Geometry check sheet. Reference: the model listing, model coordinates, mm. Give positions to 0.01 mm unless a question says otherwise; leave off trailing zeros. Write each loop counter-clockwise with the first axis right and the second up, starting at its lowest first coordinate (ties: lowest second). Pieces come first, ordered by that corner, then holes. Notation, with made-up numbers: M 0.25,10 L 40.25,10 A26 ccw 40.25,35 Z; hole C 76.25,43 d4. An arc over 180 degrees is marked long. Use one line per item in the form item = value. Start each with the question number.
Autodesk Inventor part; units mm, degrees
ref_plane "作業平面1" through (0, 0, 0) normal (0, 0, -1) x (-1, 0, 0)
ref_plane "YZ Plane" through (0, 0, 0) normal (1, 0, 0) x (0, 1, 0)
ref_plane "XZ Plane" through (0, 0, 0) normal (0, 1, 0) x (-1, 0, 0)
sketch "スケッチ1" plane through (0, 0, 0) normal (0, 0, 1) x (1, 0, 0)
  circle A0 centre (0, 0) radius 5
  circle A1 centre (0, 0) radius 4.5
  dimension "d0" = 10
  dimension "d10" = 9
ref_plane "作業平面1" through (0, 0, 0) normal (0, 0, -1) x (-1, 0, 0)
extrude "押し出し5" add sketch "スケッチ1" against normal blind 1
sketch "スケッチ3" plane through (0, 0, -1) normal (0, 0, -1) x (-1, 0, 0)
  circle A0 centre (0, 0) radius 5
extrude "押し出し6" add sketch "スケッチ3" along normal blind 59
fillet "フィレット2" radius 1 1 edges at (5, 0, -60)
properties part number "ueda_hanko_3D プリント"
(1) Sectioned sample at C-C, the plane z = -35. Record the boundary of the cut face in (x, y).
(2) Thickness scan on probe 1 along Y at (x, z) = (0, -0.3); probe 2 along Z at (x, y) = (-2.5, -1); probe 3 along X at (y, z) = (-0.25, -7.5). Record the ranges inside material, lowest first. Write a range as [from, to].
(3) Sectioned sample at A-A, the plane y = 0. Record the boundary of the cut face in (x, z).
(4) Depth check by flat-ended pin: pin 1 (2 mm diameter, centred on x = -2, z = -31.5, fed in from -Y); pin 2 (1.5 mm diameter, centred on x = 3.5, z = -15, fed in from -Y); pin 3 (3 mm diameter, centred on y = -2, z = -51.5, fed in from +X). Enter the tip coordinate at first touch or a pass-through.
(5) Draft check along Y on faces 1 (the cylindrical face through (-0.59, 4.46, -0.49)), 2 (the flat face through (0, 0, -1)), 3 (the flat face through (0, 0, -60)). Enter one of: released by +Y, released by -Y, zero draft, split by the parting line, or undercut.
Numbers:
q1.outline = C 0,0 d10
q2.probe_1 = [-5, -4.5], [4.5, 5]
q2.probe_2 = [-60, -1]
q2.probe_3 = [-4.99, 4.99]
q3.outline = M -5,-59 A1 ccw -4,-60 L 4,-60 A1 ccw 5,-59 L 5,0 L 4.5,0 L 4.5,-1 L -4.5,-1 L -4.5,0 L -5,0 Z
q4.pin_1 = -4.9
q4.pin_2 = -4.18
q4.pin_3 = 4.97
q5.face_1 = undercut
q5.face_2 = undercut
q5.face_3 = zero draft
